from build123d import *

# Parameters (mm, degrees)
F1_DEPTH      = 76.2
F1_DEPTH_BACK = 76.2


with BuildPart() as f1:
    # F0 (on Front) → F1 (new body, two sides)
    with BuildSketch(Plane.XZ) as f1_sk:
        with BuildLine():
            Line((-202.168562, 178.864715), (-202.235902, 177.8))
            Line((-202.235902, 177.8), (265.896064, 152.4))
            ThreePointArc((265.896064, 152.4), (335.923144, 159.450833), (400.48638, 187.470376))
            ThreePointArc((400.48638, 187.470376), (475.446875, 231.42442), (559.764098, 252.439644))
            Line((559.764098, 252.439644), (559.912065, 253.526855))
            ThreePointArc((559.912065, 253.526855), (475.190079, 232.471765), (399.866841, 188.340805))
            ThreePointArc((399.866841, 188.340805), (335.625955, 160.475818), (265.953862, 153.465233))
            Line((265.953862, 153.465233), (-202.168562, 178.864715))
        make_face()
    extrude(amount=F1_DEPTH)
    extrude(f1_sk.sketch, amount=-F1_DEPTH_BACK)


solid = f1.part
Source: CAD feature listing. Evaluate the final solid. Frame: model axes, mm. Round coordinates to 2 decimals unless told otherwise and drop trailing zeros. Loops run counter-clockwise (first coordinate to the right, second up) from the corner with the lowest first, then second, coordinate; pieces in that order, holes last.
Q1. Section C-C, the plane x = 444. Return loops of the section in (y, z), plus the area to 3 significant figures.
Q2. Ray query, line 1 (Z direction, x = 283, y = 38.5); line 2 (Z direction, x = 287, y = 56.5); line 3 (X direction, y = 5, z = 219). Return the intervals inside material, ascending.
Q3. Mould query, pull axis X, two halves, no side actions, for faces 1 (the face through (28.553, -1.067, 165.278)), 2 (the face through (474.32, -1.07, 230.96)), 3 (the face through (336.578, -1.067, 160.726)), 4 (the face through (35.17, -1.067, 165.987)). Classes: pulls with the +X half, pulls with the -X half, needs draft (parallel to the pull), parting line crosses it, or undercut.
Q4. First-contact query: P1, Ø2, axis at y = -3, z = 188, coming from the -X side; P2, Ø1, axis at x = 333, y = 27, coming from the +Z side; P3, Ø12, axis at y = 3, z = 195.5, coming from the +X side. Flat tips, straight axial feed; report the tip coordinate or a pass-through.
Q5. Section A-A, the plane y = -39.5. Return loops of the section in (x, z).
Q6. Section B-B, the plane z = 166. Return loops of the section in (x, y), plus the area to 3 significant figures.
Solutions:
1. outline: (-76.2, 216.45) - (76.2, 216.45) - (76.2, 217.66) - (-76.2, 217.66) - close
1. area: 185 mm2
2. line 1: z = 152.11 to 153.18
2. line 2: z = 152.23 to 153.3
2. line 3: x = 446.47 to 448.75
3. face 1: pulls with the -X half
3. face 2: pulls with the +X half
3. face 3: undercut
3. face 4: undercut
4. P1: stops at x = 397.72
4. P2: stops at z = 159.93
4. P3: stops at x = 419.55
5. outline: (-202.24, 177.8) - (265.9, 152.4) arc R228.6 ccw to (400.49, 187.47) arc R304.8 cw to (559.76, 252.44) - (559.91, 253.53) arc R305.87 ccw to (399.87, 188.34) arc R227.53 cw to (265.95, 153.47) - (-202.17, 178.86) - close
6. outline: (15.24, -76.2) - (34.93, -76.2) - (34.93, 76.2) - (15.24, 76.2) - close; (353.72, -76.2) - (356.88, -76.2) - (356.88, 76.2) - (353.72, 76.2) - close
6. area: 3,480 mm2
